Work out the finished part from the listing and answer in its coordinate system (mm). Face numbers are marked on the shaded views. A direction names the side the tool comes from. Give positions to 0.01 mm unless a question says otherwise; leave off trailing zeros. Order: outer loops, then holes, each group sorted by start corner. A loop starts at its lowest first (then second) coordinate and runs counter-clockwise, first axis right, second up. Notation, with made-up numbers: (-4, 48.25) - (47, 48.25) arc R27 cw to (47, 68.25) - close; hole circle Ø8 at (34, -28). An arc over 180 degrees is marked (long way). Return JSON: item names as keys, results as strings. Group by question number.
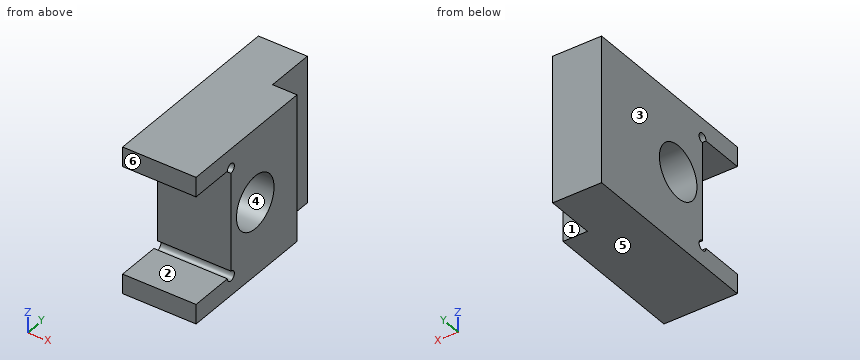
from build123d import *

# Parameters (mm, degrees)
RESSALTO_EXTRUS_O1_DEPTH = 30
ESBO_O2_W                = 22
ESBO_O2_H                = 10
CORTE_EXTRUS_O1_DEPTH    = 52.439284598
ESBO_O3_R                = 1
CORTE_EXTRUS_O2_DEPTH    = 52.439284598
ESBO_O4_R                = 5.395012771
CORTE_EXTRUS_O3_DEPTH    = 52.439284598


with BuildPart() as part:
    # Esboço1 → Ressalto-extrusão1 (new body)
    with BuildSketch(Plane.XY):
        Polygon((0, 0), (0, -39), (15, -39), (15, -10), (10, -10), (10, 0), align=None)
    extrude(amount=RESSALTO_EXTRUS_O1_DEPTH)

    # Esboço2 → Corte-extrusão1 (cut, through all)
    with BuildSketch(Plane(origin=(15, 0, 0), x_dir=(0, 0, -1), z_dir=(1, 0, 0))):
        with Locations((-15, -34)):
            Rectangle(ESBO_O2_W, ESBO_O2_H)
    extrude(amount=-CORTE_EXTRUS_O1_DEPTH, mode=Mode.SUBTRACT)

    # Esboço3 → Corte-extrusão2 (cut, through all)
    with BuildSketch(Plane(origin=(15, 0, 0), x_dir=(0, 0, -1), z_dir=(1, 0, 0))):
        with Locations((-26, -29)):
            Circle(ESBO_O3_R)
        with Locations((-4, -29)):
            Circle(ESBO_O3_R)
    extrude(amount=-CORTE_EXTRUS_O2_DEPTH, mode=Mode.SUBTRACT)

    # Esboço4 → Corte-extrusão3 (cut, through all)
    with BuildSketch(Plane(origin=(15, 0, 0), x_dir=(0, 0, -1), z_dir=(1, 0, 0))):
        with Locations(Location((-15, -22, 0), (0, 0, 90))):
            Circle(ESBO_O4_R)
    extrude(amount=-CORTE_EXTRUS_O3_DEPTH, mode=Mode.SUBTRACT)


solid = part.part
1. The part is cut by section C-C (x = 7.75). Give the vertices of the cut face in (y, z), and give its area (3 significant figures).
2. Consider probe 1 along Z at (x, y) = (11.75, -28.5); probe 2 along Z at (x, y) = (5.75, -36); probe 3 along Y at (x, z) = (11.5, 8.5). Determine where each line is inside the solid, lowest interval first. Write a range as from..to.
3. Determine the mould class of the marked faces 4, 5 and 6 for opening direction Z: released by +Z, released by -Z, zero draft, split by the parting line, or undercut.
4. The part is cut by section A-A (z = 15). Give the vertices of the cut face in (x, y), and give its area (3 significant figures).
5. Each of these flat-tipped pins is pushed along its axis until it touches: pin 1 (6.5 mm diameter, centred on y = -22, z = 15, fed in from -X); pin 2 (5 mm diameter, centred on y = -4, z = 16.5, fed in from +X); pin 3 (1.5 mm diameter, centred on x = 13, z = 19.5, fed in from -Y); pin 4 (2.5 mm diameter, centred on x = 13, z = 7.5, fed in from +Y). Where does it stop, or does it pass through?
6. The part is cut by section D-D (z = 11). Give the vertices of the cut face in (x, y), and give its area (3 significant figures).
7. A tool of negligible diameter and unlimited length cuts with its end or side. For the marked faces 1, 2 and 3, from which of +Z, -Z, +X, -X, +Y, -Y can it reach the whole face along a straight path? Write none if from no direction.
8. The part is cut by section B-B (y = -22). Give the vertices of the cut face in (x, z).
Answers:
{
 "1": {"outline": "(-39, 0) - (0, 0) - (0, 30) - (-39, 30) - (-39, 26) - (-30, 26) arc R1 cw (long way) to (-29, 25) - (-29, 5) arc R1 cw (long way) to (-30, 4) - (-39, 4) - close; hole circle Ø10.79 at (-22, 15)", "area": "854 mm^2"},
 "2": {"probe 1": "z = 0..3.13, 4.87..25.13, 26.87..30", "probe 2": "z = 0..4, 26..30", "probe 3": "y = -29..-10"},
 "3": {"face 4": "undercut", "face 5": "released by -Z", "face 6": "zero draft"},
 "4": {"outline": "(0, -29) - (15, -29) - (15, -27.4) - (0, -27.4) - close; (0, -16.6) - (15, -16.6) - (15, -10) - (10, -10) - (10, 0) - (0, 0) - close", "area": "223 mm^2"},
 "5": {"pin 1": "passes through", "pin 2": "stops at x = 10", "pin 3": "stops at y = -29", "pin 4": "stops at y = -10"},
 "6": {"outline": "(0, -29) - (15, -29) - (15, -25.62) - (0, -25.62) - close; (0, -18.38) - (15, -18.38) - (15, -10) - (10, -10) - (10, 0) - (0, 0) - close", "area": "276 mm^2"},
 "7": {"face 1": "+Z, -Z, +X, +Y", "face 2": "+X, -X, -Y", "face 3": "+Z, -Z, -X, +Y, -Y"},
 "8": {"outline": "(0, 0) - (15, 0) - (15, 9.6) - (0, 9.6) - close; (0, 20.4) - (15, 20.4) - (15, 30) - (0, 30) - close"}
}
